Build history of the part. All positions in model axes, mm. A direction names the side the tool comes from. Coordinates: 2 decimals unless noted, no trailing zeros. Order: outer loops, then holes, each group sorted by start corner. A loop starts at its lowest first (then second) coordinate and runs counter-clockwise, first axis right, second up. Notation, with made-up numbers: (14.5, 84) - (44.5, 84) arc R19 cw to (44.5, 119) - close; hole circle Ø2 at (-18, 33). An arc over 180 degrees is marked (long way). Return JSON: item names as keys, results as strings.
from build123d import *

# Parameters (mm, degrees)
F0_R     = 19.05
F1_DEPTH = 101.6
F0_W     = 50.8
F0_H     = 50.8
F2_DEPTH = 50.8
F3_R     = 19.05
F4_DEPTH = 50.8
F5_R     = 19.05
F6_DEPTH = 50.8
F7_R     = 2.54
F8_R     = 2.54


with BuildPart() as f1:
    # F0 (on Front) → F1 (new body)
    with BuildSketch(Plane.XZ):
        with Locations((25.4, 25.4)):
            Circle(F0_R)
    extrude(amount=F1_DEPTH)

    # F0 (on Front) → F2 (join)
    with BuildSketch(Plane.XZ):
        with Locations((25.4, 25.4)):
            Rectangle(F0_W, F0_H)
        with Locations((25.4, 25.4)):
            Circle(F0_R, mode=Mode.SUBTRACT)
    extrude(amount=F2_DEPTH)

    # F3 (on face) → F4 (join)
    with BuildSketch(Plane.XY.offset(50.8)):
        with Locations((25.4, -25.4)):
            Circle(F3_R)
    extrude(amount=F4_DEPTH)

    # F5 (on face) → F6 (join)
    with BuildSketch(Plane(origin=(0, 0, 0), x_dir=(-1, 0, 0), z_dir=(0, 1, 0))):
        with Locations((-25.4, 25.4)):
            Circle(F5_R)
    extrude(amount=F6_DEPTH)

    # F7
    f7_edges = [f1.edges().sort_by_distance(p)[0] for p in [
        (25.4, -50.8, 50.8),
        (50.8, -25.4, 50.8),
        (25.4, 0, 50.8),
        (0, -25.4, 50.8),
    ]]
    fillet(f7_edges, radius=F7_R)

    # F8
    f8_edges = [f1.edges().sort_by_distance(p)[0] for p in [
        (50.8, -25.4, 0),
        (25.4, -50.8, 0),
        (25.4, 0, 0),
        (0, -25.4, 0),
    ]]
    fillet(f8_edges, radius=F8_R)


solid = f1.part
1. Drop flat-ended pins along their axis: pin 1 (10 mm diameter, centred on x = 36.5, z = 71.5, fed in from +Y); pin 2 (6 mm diameter, centred on x = 11, y = -76.5, fed in from +Z); pin 3 (12 mm diameter, centred on x = 20, y = 13, fed in from -Z). Give the stop position or say it passes through.
Check values:
{"pin 1": "y = -7.35", "pin 2": "z = 40.66", "pin 3": "z = 6.35"}
2. Cut at C-C on z = 25.4. Give the cut face in (x, y).
Check values:
{"outline": "(0, -50.8) - (6.35, -50.8) - (6.35, -101.6) - (44.45, -101.6) - (44.45, -50.8) - (50.8, -50.8) - (50.8, 0) - (44.45, 0) - (44.45, 50.8) - (6.35, 50.8) - (6.35, 0) - (0, 0) - close"}
3. Cut at A-A on x = 46. Give the cut face in (y, z).
Check values:
{"outline": "(-50.8, 2.54) arc R2.54 ccw to (-48.26, 0) - (-2.54, 0) arc R2.54 ccw to (0, 2.54) - (0, 48.26) arc R2.54 ccw to (-2.54, 50.8) - (-48.26, 50.8) arc R2.54 ccw to (-50.8, 48.26) - close"}
4. Tool access for faces 1 (the flat face through (25, -101.6, 26)), 2 (the cylindrical face through (21.27, -75.844, 6.803)), 3 (the cylindrical face through (11.359, -12.525, 75.844)), 4 (the flat face through (14, 0, 41)), 5 (the flat face through (25, -25, 101.6)): list every direction of +Z, -Z, +X, -X, +Y, -Y with a clear straight run to the whole face (end or side of a thin tool).
Check values:
{"face 1": "+Z, -Z, +X, -X, -Y", "face 2": "-Y", "face 3": "+Z", "face 4": "+Y", "face 5": "+Z, +X, -X, +Y, -Y"}
5. Cut at D-D on x = 25.4. Give the cut face in (y, z), plus the area to 3 significant figures.
Check values:
{"outline": "(-101.6, 6.35) - (-50.8, 6.35) - (-50.8, 2.54) arc R2.54 ccw to (-48.26, 0) - (-2.54, 0) arc R2.54 ccw to (0, 2.54) - (0, 6.35) - (50.8, 6.35) - (50.8, 44.45) - (0, 44.45) - (0, 48.26) arc R2.54 ccw to (-2.54, 50.8) - (-6.35, 50.8) - (-6.35, 101.6) - (-44.45, 101.6) - (-44.45, 50.8) - (-48.26, 50.8) arc R2.54 ccw to (-50.8, 48.26) - (-50.8, 44.45) - (-101.6, 44.45) - close", "area": "8,380 mm²"}
6. Probe L1, parallel to Y at x = 47.5, z = 15.5; L2, parallel to Y at x = 25, z = 87.5; L3, parallel to Z at x = 25.5, y = 13. List the from-to ranges inside material, lowest first.
Check values:
{"L1": "-50.8 to 0", "L2": "-44.45 to -6.35", "L3": "6.35 to 44.45"}
7. Cut at B-B on y = -25.4. Give the cut face in (x, z).
Check values:
{"outline": "(0, 2.54) arc R2.54 ccw to (2.54, 0) - (48.26, 0) arc R2.54 ccw to (50.8, 2.54) - (50.8, 48.26) arc R2.54 ccw to (48.26, 50.8) - (44.45, 50.8) - (44.45, 101.6) - (6.35, 101.6) - (6.35, 50.8) - (2.54, 50.8) arc R2.54 ccw to (0, 48.26) - close"}
